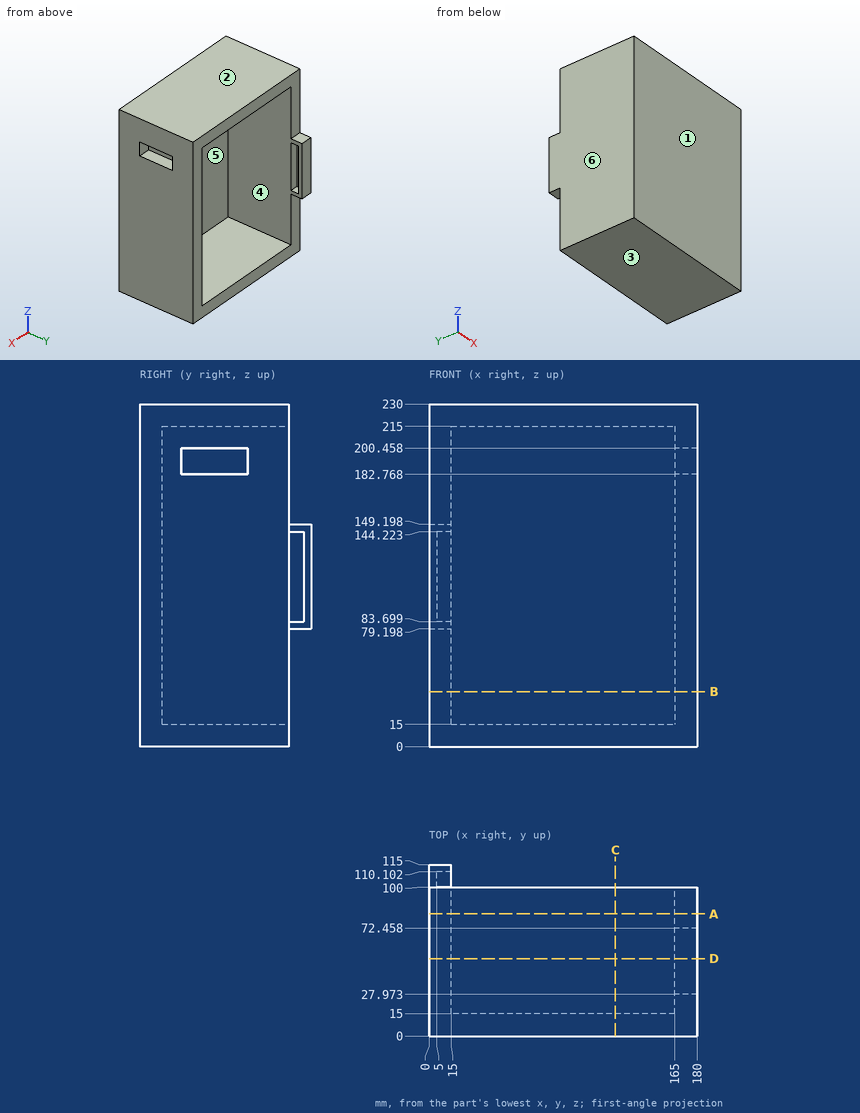
Could you check a few things on this drawing? It's one solid part, dimensions in mm from its lowest x, y, z. A direction names the side the tool comes from. Coordinates: 2 decimals unless noted, no trailing zeros. Order: outer loops, then holes, each group sorted by start corner. A loop starts at its lowest first (then second) coordinate and runs counter-clockwise, first axis right, second up. Notation, with made-up numbers: M -8.75,-2 L 12.25,-2 A20 cw 12.25,37 Z; hole C -11,48 d8. An arc over 180 degrees is marked long. Answer as a JSON object with one key per item and string values. Group by question number.
(1) Suppose I cut it at D-D, the plane y = 52. Please give me the cut outline in (x, z).
(2) Suppose I cut it at C-C, the plane x = 125. Please give me the cut outline in (y, z), then the cut area to 3 significant figures.
(3) If we mould it in two halves opening along Z, with no side actions, what happens to the marked faces 1, 2, 3 and 4? For each: released by +Z, released by -Z, zero draft, split by the parting line, or undercut.
(4) I need wall thicknesses on probe 1 along X at (y, z) = (22.5, 123.5); probe 2 along Z at (x, y) = (19.5, 65); probe 3 along Y at (x, z) = (167.5, 194.5). Which ranges of each line are inside material? Lowest first, please.
(5) Suppose I cut it at B-B, the plane z = 37. Please give me the cut outline in (x, y), then the cut area to 3 significant figures.
(6) For pin 1 (4.5 mm diameter, centred on x = 173, z = 194, fed in from +Y); pin 2 (5 mm diameter, centred on x = 83, z = 92.5, fed in from +Y); pin 3 (4.5 mm diameter, centred on x = 10.5, y = 110.5, fed in from +Z), each with a flat end and sliding along its axis, tell me the tip position at first contact or that it passes through.
(7) Suppose I cut it at A-A, the plane y = 82. Please give me the cut outline in (x, z), then the cut area to 3 significant figures.
(8) Which directions (+Z, -Z, +X, -X, +Y, -Y) give clear straight access to the entire face, cutting with the end or side of a thin tool? Please do the marked faces 5 and 6.
Values found:
{
 "1": {"outline": "M 0,0 L 180,0 L 180,182.77 L 165,182.77 L 165,15 L 15,15 L 15,215 L 165,215 L 165,200.46 L 180,200.46 L 180,230 L 0,230 Z"},
 "2": {"outline": "M 0,0 L 100,0 L 100,15 L 15,15 L 15,215 L 100,215 L 100,230 L 0,230 Z", "area": "6,000 mm^2"},
 "3": {"face 1": "zero draft", "face 2": "released by +Z", "face 3": "released by -Z", "face 4": "undercut"},
 "4": {"probe 1": "x = 0 to 15, 165 to 180", "probe 2": "z = 0 to 15, 215 to 230", "probe 3": "y = 0 to 27.97, 72.46 to 100"},
 "5": {"outline": "M 0,0 L 180,0 L 180,100 L 165,100 L 165,15 L 15,15 L 15,100 L 0,100 Z", "area": "5,250 mm^2"},
 "6": {"pin 1": "stops at y = 100", "pin 2": "stops at y = 15", "pin 3": "stops at z = 149.2"},
 "7": {"outline": "M 0,0 L 180,0 L 180,230 L 0,230 Z; hole M 15,15 L 165,15 L 165,215 L 15,215 Z", "area": "11,400 mm^2"},
 "8": {"face 5": "+Y", "face 6": "+Z, -Z, -X, +Y, -Y"}
}
